The model under review builds one solid part; all positions refer to its coordinate system, in mm. Face numbers are marked on the shaded views. Coordinates: 2 decimals unless noted, no trailing zeros. Loops run counter-clockwise (first coordinate to the right, second up) from the corner with the lowest first, then second, coordinate; pieces in that order, holes last. Notation, with made-up numbers: (17, -27) - (45, -27) arc R14 cw to (45, -22) - close; hole circle Ø4 at (89, 40). An arc over 180 degrees is marked (long way). Use a Markdown table: item, result. Add a question column.
1) Add section B-B, the plane x = 0. Give the boundary of the cut face in (y, z), and give its area (3 significant figures).
2) The part is to be moulded in two halves that separate along Y. For the marked faces 1, 2 and 3, say which applies: pulls with the +Y half, pulls with the -Y half, needs draft (parallel to the pull), parting line crosses it, or undercut.
3) Add section D-D, the plane y = 6. Give the boundary of the cut face in (x, z), and give its area (3 significant figures).
4) Add section A-A, the plane z = 3.6. Give the number of separate pieces and of enclosed holes in the cut face, and give its area (3 significant figures).
5) To check wall thickness, follow L1, parallel to Y at x = 12, z = 1.9; L2, parallel to Y at x = 0, z = 4.25; L3, parallel to Y at x = -6, z = 3.3. State the ranges of each line that lie inside material, in increasing order. Write a range as [from, to].
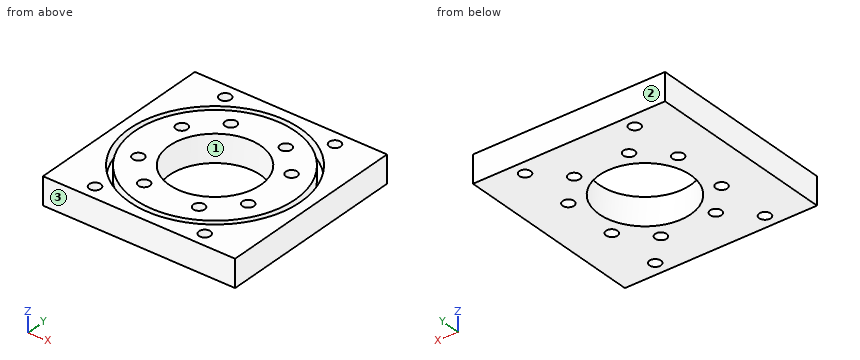
```python
from build123d import *

# Parameters (mm, degrees)
SKETCH_1_W          = 42
SKETCH_1_H          = 42
SKETCH_1_R          = 1.25
SKETCH_1_R_2        = 10
EXTRUDE_1_DEPTH     = 6
SKETCH_2_R          = 18.7
SKETCH_2_R_2        = 17.5
CUT_EXTRUDE_1_DEPTH = 3


with BuildPart() as part:
    # 草圖1 → 填料-伸長1 (new body)
    with BuildSketch(Plane.XY):
        Rectangle(SKETCH_1_W, SKETCH_1_H)
        with Locations((-6, 12)):
            Circle(SKETCH_1_R, mode=Mode.SUBTRACT)
        with Locations((-12, 6)):
            Circle(SKETCH_1_R, mode=Mode.SUBTRACT)
        with Locations((-12, -6)):
            Circle(SKETCH_1_R, mode=Mode.SUBTRACT)
        with Locations((-6, -12)):
            Circle(SKETCH_1_R, mode=Mode.SUBTRACT)
        with Locations((6, 12)):
            Circle(SKETCH_1_R, mode=Mode.SUBTRACT)
        with Locations((12, 6)):
            Circle(SKETCH_1_R, mode=Mode.SUBTRACT)
        with Locations((12, -6)):
            Circle(SKETCH_1_R, mode=Mode.SUBTRACT)
        with Locations((6, -12)):
            Circle(SKETCH_1_R, mode=Mode.SUBTRACT)
        with Locations((-12, 18)):
            Circle(SKETCH_1_R, mode=Mode.SUBTRACT)
        with Locations((12, 18)):
            Circle(SKETCH_1_R, mode=Mode.SUBTRACT)
        with Locations((-12, -18)):
            Circle(SKETCH_1_R, mode=Mode.SUBTRACT)
        with Locations((12, -18)):
            Circle(SKETCH_1_R, mode=Mode.SUBTRACT)
        Circle(SKETCH_1_R_2, mode=Mode.SUBTRACT)
    extrude(amount=EXTRUDE_1_DEPTH)

    # 草圖2 → 除料-伸長1 (cut)
    with BuildSketch(Plane.XY.offset(6)):
        Circle(SKETCH_2_R)
        Circle(SKETCH_2_R_2, mode=Mode.SUBTRACT)
    extrude(amount=-CUT_EXTRUDE_1_DEPTH, mode=Mode.SUBTRACT)


solid = part.part
```
From the geometry:
| question | item | result |
|---|---|---|
| 1 | outline | (-21, 0) - (-10, 0) - (-10, 6) - (-17.5, 6) - (-17.5, 3) - (-18.7, 3) - (-18.7, 6) - (-21, 6) - close; (10, 0) - (21, 0) - (21, 6) - (18.7, 6) - (18.7, 3) - (17.5, 3) - (17.5, 6) - (10, 6) - close |
| 1 | area | 125 mm^2 |
| 2 | face 1 | undercut |
| 2 | face 2 | pulls with the +Y half |
| 2 | face 3 | pulls with the -Y half |
| 3 | outline | (-21, 0) - (-13.25, 0) - (-13.25, 6) - (-16.44, 6) - (-16.44, 3) - (-17.71, 3) - (-17.71, 6) - (-21, 6) - close; (-10.75, 0) - (-8, 0) - (-8, 6) - (-10.75, 6) - close; (8, 0) - (10.75, 0) - (10.75, 6) - (8, 6) - close; (13.25, 0) - (21, 0) - (21, 6) - (17.71, 6) - (17.71, 3) - (16.44, 3) - (16.44, 6) - (13.25, 6) - close |
| 3 | area | 118 mm^2 |
| 4 | separate pieces | 2 |
| 4 | enclosed holes | 14 |
| 4 | area | 1,250 mm^2 |
| 5 | L1 | y = [-21, -19.25], [-16.75, -7.25], [-4.75, 4.75], [7.25, 16.75], [19.25, 21] |
| 5 | L2 | y = [-21, -18.7], [-17.5, -10], [10, 17.5], [18.7, 21] |
| 5 | L3 | y = [-21, -17.71], [-16.44, -13.25], [-10.75, -8], [8, 10.75], [13.25, 16.44], [17.71, 21] |
